Here's how the part is built. I have some questions about the finished solid (model axes, mm). Face numbers are marked on the shaded views. A direction names the side the tool comes from. Give positions to 0.01 mm unless a question says otherwise; leave off trailing zeros. Order: outer loops, then holes, each group sorted by start corner. A loop starts at its lowest first (then second) coordinate and runs counter-clockwise, first axis right, second up.
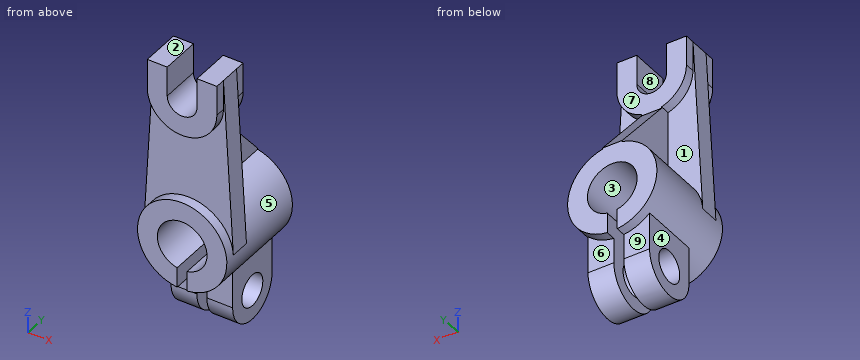
Autodesk Inventor part; units mm, degrees
ref_plane "YZ Plane" through (0, 0, 0) normal (1, 0, 0) x (0, 1, 0)
ref_plane "XZ Plane" through (0, 0, 0) normal (0, 1, 0) x (-1, 0, 0)
ref_plane "XY Plane" through (0, 0, 0) normal (0, 0, 1) x (1, 0, 0)
sketch "Náčrt3" plane through (0, 0, 0) normal (0, 1, 0) x (-1, 0, 0)
  line L0 (18.7116, 64.0709) -> (8.7116, 64.0709)
  line L1 (8.7116, 64.0709) -> (8.7116, 49.0709)
  arc A0 (-6.2884, 49.0709) -> (8.7116, 49.0709) centre (1.2116, 49.0709) ccw
  line L2 (-6.2884, 49.0709) -> (-6.2884, 64.0709)
  line L3 (-6.2884, 64.0709) -> (-16.2884, 64.0709)
  arc A1 (3.6769, -38.1765) -> (-1.3231, -38.1765) centre (1.1769, -25.9291) ccw
  arc A2 (3.6769, -48.2898) -> (-1.3231, -48.2898) centre (1.1769, -25.9291) ccw
  line L4 (18.7116, 64.0709) -> (23.6423, -24.681)
  line L5 (-16.2884, 64.0709) -> (-21.2875, -24.6635)
  arc A3 (-16.2884, 49.0709) -> (18.7116, 49.0709) centre (1.2116, 49.0709) ccw
  line L6 (18.7116, 49.0709) -> (18.7116, 64.0709)
  line L7 (-16.2884, 49.0709) -> (-16.2884, 64.0709)
  line L8 (-1.3231, -38.1765) -> (-1.3231, -48.2898)
  line L9 (3.6769, -48.2898) -> (3.6769, -38.1765)
  point P0 (0, 0)
  dimension "d0" = 10
  dimension "d1" = 10
  dimension "d2" = 15
  dimension "d3" = 15
  dimension "d4" = 7.5
  dimension "d5" = 25
  dimension "d6" = 45
  dimension "d7" = 75
  dimension "d11" = 3.18
  dimension "d12" = 22.2368
  dimension "d13" = 18.7116
  dimension "d16" = 15.0347
  dimension "d17" = 20.0347
extrude "Vysunutí1" add sketch "Náčrt3" against normal blind 5 contours L6 A3 L7 L3 L2 A0 L1 L0 | A2 L9 A1 L8
extrude "Vysunutí2" add sketch "Náčrt3" along normal blind 10 contours L4 A2 L5 L7 A3 L6
extrude "Vysunutí3" add sketch "Náčrt3" along normal blind 15 contours L6 A3 L7 L3 L2 A0 L1 L0
extrude "Vysunutí4" add sketch "Náčrt3" along normal blind 45 contours A2 L9 A1 L8
ref_plane "Pracovní rovina1" through (-1.3339, 0, 376.8696) normal (1, 0, 0.0004) x (0, 1, 0)
sketch "Náčrt4" plane through (-1.3339, 0, 376.8696) normal (1, 0, 0.0004) x (0, 1, 0)
  line L0 (45, -425.1604) -> (45, -380.2987)
  line L1 (15, -345.2987) -> (45, -380.2987)
  line L2 (45, -380.2987) -> (45, -385.2987)
  line L3 (45, -385.2987) -> (10, -385.2987)
  line L4 (10, -401.5419) -> (10, -312.7919)
  line L5 (15, -345.2987) -> (15, -327.7919)
  line L6 (10, -345.2987) -> (10, -385.2987)
  line L7 (15, -345.2987) -> (15, -343.2987)
  line L8 (15, -343.2987) -> (10, -343.2987)
  line L9 (10, -327.7919) -> (10, -345.2987)
  line L10 (15, -343.2987) -> (10, -343.2987)
  line L11 (10, -345.2987) -> (10, -343.2987)
  point P0 (0, -376.8701)
  point P1 (45, -425.1584)
  point P2 (15, -327.8055)
  point P3 (10, -327.8055)
  dimension "d26" = 5
  dimension "d28" = 42
extrude "Vysunutí5" add sketch "Náčrt4" along normal blind 5
extrude "Vysunutí6" add sketch "Náčrt4" against normal blind 5
sketch "Náčrt7" plane through (-3.6769, -5, -38.1765) normal (1, 0, 0) x (0, 0, -1)
  line L0 (0, 15) -> (10.2526, 15)
  line L1 (10.2526, 15) -> (22.7526, 15)
  line L2 (22.7526, 45) -> (0, 45)
  line L3 (0, 45) -> (0, 15)
  arc A0 (22.7526, 15) -> (22.7526, 45) centre (22.7526, 30) ccw
  circle A1 centre (22.7526, 30) radius 8
  point P0 (-38.1765, 5)
  dimension "d45" = 12.5
  dimension "d46" = 30
  dimension "d47" = 16
  dimension "d48" = 10
  dimension "d49" = 38.1765
  dimension "d50" = 22.7525
extrude "Vysunutí7" add sketch "Náčrt7" along normal blind 18
extrude "Vysunutí8" cut sketch "Náčrt7" along normal blind 5
extrude "Vysunutí9" add sketch "Náčrt7" against normal blind 13
properties part number "2"
Q1. If we section it at A-A on x = -10: List the corners of the cut face in (y, z) for me.
Filled sheet:
outline: (-5, -46.63) - (10, -46.63) - (10, -60.93) arc R15 ccw to (40, -60.93) - (40, -46.63) - (45, -46.63) - (45, -34.78) - (-5, -34.78) - close; (-5, -17.07) - (45, -17.07) - (45, -5.23) - (10, -5.23) - (10, 33.94) - (15, 33.94) - (15, 64.07) - (-5, 64.07) - (-5, 33.94) - (0, 33.94) - (0, -5.23) - (-5, -5.23) - close; hole circle Ø16 at (25, -60.93)
Q2. If we section it at B-B on y = 25: List the corners of the cut face in (x, z) for me, plus the area to 3 significant figures.
Filled sheet:
outline: (-16.68, -75.93) - (-3.68, -75.93) - (-3.68, -68.93) - (-16.68, -68.93) - close; (-16.68, -52.93) - (-3.68, -52.93) - (-3.68, -38.18) arc R12.5 cw (long way) to (1.32, -38.18) - (1.32, -52.93) - (14.32, -52.93) - (14.32, -42.24) arc R22.5 ccw to (3.82, -3.99) - (3.81, 19.91) - (-6.19, 19.9) - (-6.18, -3.99) arc R22.5 ccw to (-16.68, -42.24) - close; (1.32, -75.93) - (14.32, -75.93) - (14.32, -68.93) - (1.32, -68.93) - close
area: 1,640 mm2
Q3. For the marked faces 5, 6, 7, 8 and 9, which set-ups out of +Z, -Z, +X, -X, +Y, -Y let a thin tool reach every point of the face, with its end or its side?
Filled sheet:
face 5: none
face 6: -Z, +X, +Y
face 7: +Z, +X, -X, +Y
face 8: +Z, +Y, -Y
face 9: -Z, -X, +Y
Q4. Thinking about a two-plate mould opening in Z: for the marked faces 1, 2, 3 and 4, which applies, released by +Z, released by -Z, zero draft, split by the parting line, or undercut?
Filled sheet:
face 1: undercut
face 2: released by +Z
face 3: undercut
face 4: zero draft
Q5. I need wall thicknesses on L1, parallel to X at y = 39.5, z = -26.5; L2, parallel to X at y = 34.5, z = 5.5; L3, parallel to X at y = 35.5, z = -69. Which ranges of each line are inside material? Lowest first, please.
Filled sheet:
L1: x = -23.67 to -13.66, 11.31 to 21.32
L2: x = -6.19 to 3.81
L3: x = -16.68 to -3.68, 1.32 to 14.32
Q6. I'm going to push flat-ended pins straight in: P1, Ø12, axis at x = -14, y = 15.5, coming from the +Z side; P2, Ø1.5, axis at x = 9, z = -28.5, coming from the -Y side; P3, Ø12, axis at y = 7, z = 60.5, coming from the -X side; P4, Ø6.5, axis at x = 8, z = -56, coming from the -Y side. Where does each tip first touch, or does it pass through?
Filled sheet:
P1: stops at z = 64.07
P2: passes through
P3: stops at x = -19.24
P4: stops at y = 10
Q7. If we section it at C-C on z = 44: List the corners of the cut face in (x, y) for me.
Filled sheet:
outline: (-19.83, 0) - (-17.96, 0) - (-17.96, -5) - (-6.74, -5) - (-6.74, 15) - (-17.96, 15) - (-17.96, 10) - (-19.83, 10) - close; (4.31, -5) - (15.54, -5) - (15.54, 0) - (17.42, 0) - (17.42, 10) - (15.54, 10) - (15.54, 15) - (4.31, 15) - close
Q8. If we section it at D-D on y = 5: List the corners of the cut face in (x, z) for me, plus the area to 3 significant figures.
Filled sheet:
outline: (-23.64, -24.68) arc R22.5 ccw to (-3.68, -48.29) - (-3.68, -38.18) arc R12.5 cw (long way) to (1.32, -38.18) - (1.32, -48.29) arc R22.5 ccw to (21.29, -24.66) - (16.29, 64.07) - (6.29, 64.07) - (6.29, 49.07) arc R7.5 cw to (-8.71, 49.07) - (-8.71, 64.07) - (-18.71, 64.07) - close
area: 3,540 mm2
